Verification items for the finished model (mm, model axes). A direction names the side the tool comes from. Coordinates: 2 decimals unless noted, no trailing zeros. Order: outer loops, then holes, each group sorted by start corner. A loop starts at its lowest first (then second) coordinate and runs counter-clockwise, first axis right, second up. Notation, with made-up numbers: M 66.25,50.25 L 116.25,50.25 A19 ccw 116.25,82.25 Z; hole C 81.5,-26 d11. An arc over 180 degrees is marked long. Return JSON: item names as keys, results as strings.
```python
from build123d import *

# Parameters (mm, degrees)
SKETCH2_W           = 50.8
SKETCH2_H           = 38.1
BOSS_EXTRUDE1_DEPTH = 12.7
FILLET1_R           = 6.35
SKETCH3_R           = 3.81
CUT_EXTRUDE1_DEPTH  = 35.195796525
SKETCH7_W           = 12.7
SKETCH7_H           = 12.7
BOSS_EXTRUDE2_DEPTH = 19.05
SKETCH8_R           = 5.08
CUT_EXTRUDE2_DEPTH  = 25.4
SKETCH9_W           = 6.35
SKETCH9_H           = 38.1
CUT_EXTRUDE3_DEPTH  = 44.45
CUT_EXTRUDE4_REACH  = 52
SKETCH10_W          = 6.35
SKETCH10_H          = 6.35
CHAMFER6_SIZE       = 17.78
CHAMFER6_SIZE_2     = 12.449690029


with BuildPart() as part:
    # Sketch2 → Boss-Extrude1 (new body)
    with BuildSketch(Plane.XY):
        Rectangle(SKETCH2_W, SKETCH2_H)
    extrude(amount=BOSS_EXTRUDE1_DEPTH)

    # Fillet1
    fillet1_edges = [part.edges().sort_by_distance(p)[0] for p in [
        (-25.4, 19.05, 6.35),
        (25.4, 19.05, 6.35),
        (-25.4, -19.05, 6.35),
    ]]
    fillet(fillet1_edges, radius=FILLET1_R)

    # Sketch3 → Cut-Extrude1 (cut, through all)
    with BuildSketch(Plane.XY.offset(12.7)):
        with Locations((-6.35, -10.16)):
            Circle(SKETCH3_R)
    extrude(amount=-CUT_EXTRUDE1_DEPTH, mode=Mode.SUBTRACT)

    # Sketch7 → Boss-Extrude2 (add)
    with BuildSketch(Plane(origin=(25.4, 0, 0), x_dir=(0, 0, -1), z_dir=(1, 0, 0))):
        with Locations((-6.35, 6.35)):
            Rectangle(SKETCH7_W, SKETCH7_H)
    extrude(amount=BOSS_EXTRUDE2_DEPTH)

    # Sketch8 → Cut-Extrude2 (cut)
    with BuildSketch(Plane(origin=(44.45, 0, 0), x_dir=(0, 0, -1), z_dir=(1, 0, 0))):
        with Locations((-6.35, 6.35)):
            Circle(SKETCH8_R)
    extrude(amount=-CUT_EXTRUDE2_DEPTH, mode=Mode.SUBTRACT)

    # Sketch9 → Cut-Extrude3 (cut)
    with BuildSketch(Plane.ZY.offset(25.4)):
        with Locations((3.175, 0)):
            Rectangle(SKETCH9_W, SKETCH9_H)
    extrude(amount=-CUT_EXTRUDE3_DEPTH, mode=Mode.SUBTRACT)

    # Sketch10 → Cut-Extrude4 (cut, up to next)
    with BuildSketch(Plane.ZY.offset(-19.05), mode=Mode.PRIVATE) as cut_extrude4_sk1:
        with Locations((3.175, -15.875)):
            Rectangle(SKETCH10_W, SKETCH10_H)
    cut_extrude4_tool1 = extrude(cut_extrude4_sk1.sketch, amount=-CUT_EXTRUDE4_REACH, mode=Mode.PRIVATE) & part.part
    add(cut_extrude4_tool1.solids().sort_by_distance((19.05, -15.875, 3.175))[0], mode=Mode.SUBTRACT)

    # Chamfer6
    # the kernel refuses this chamfer: 17.78, 12.449690029 mm, written as the material it takes off along each edge
    with BuildSketch(Plane(origin=(25.4, -19.05, -39.567778654), x_dir=(-0.9997533347641299, -0.022209674198457294, 0), z_dir=(0, 0, 1))) as chamfer6_piece_1:
        Polygon((CHAMFER6_SIZE * 0.999753334764, -CHAMFER6_SIZE * 0.0222096741985), (-CHAMFER6_SIZE_2 * 0.0222096741991, -CHAMFER6_SIZE_2 * 0.999753334794), (0, 0), align=None)
    extrude(amount=98.185557309, mode=Mode.SUBTRACT)


solid = part.part
```
Q1. Go/stop test with flat-tipped pins: pin 1 (1.5 mm diameter, centred on y = 4.5, z = 5.5, fed in from -X); pin 2 (3 mm diameter, centred on y = 2.5, z = 2.5, fed in from -X); pin 3 (19 mm diameter, centred on x = -3, y = 4, fed in from -Z); pin 4 (4 mm diameter, centred on x = 34.5, z = 7, fed in from -Y). Record where each tip stops, or that it passes through.
Values:
{"pin 1": "through", "pin 2": "x = 19.05", "pin 3": "z = 6.35", "pin 4": "y = 0"}
Q2. Material ranges on line 1 along Y through (x, z) = (31.5, 6.35); line 2 along X through (y, z) = (-3, 2), recorded low to high.
Values:
{"line 1": "0 to 1.27, 11.43 to 12.7", "line 2": "19.05 to 25.4"}
Q3. Cross-section at B-B, the plane x = -6.35. Record the boundary of the cut face in (y, z), and give its area (3 significant figures).
Values:
{"outline": "M -19.05,6.35 L -13.97,6.35 L -13.97,12.7 L -19.05,12.7 Z; M -6.35,6.35 L 19.05,6.35 L 19.05,12.7 L -6.35,12.7 Z", "area": "194 mm^2"}
Q4. Tool access check on faces 4 (the face through (35, 0, 6)), 5 (the face through (19.05, 6, 8)), 6 (the face through (35, 12.7, 6)), 7 (the face through (-3, 0, 6.35)). Record the directions out of +Z, -Z, +X, -X, +Y, -Y that give a thin tool (end or side, any length) a straight path to the whole face; none if there is none.
Values:
{"face 4": "+Z, -Z, +X, -Y", "face 5": "+X", "face 6": "+Z, -Z, +X, +Y", "face 7": "-Z, -X, +Y, -Y"}
Q5. Cross-section at C-C, the plane z = 3.5. Record the boundary of the cut face in (x, y), and give its area (3 significant figures).
Values:
{"outline": "M 19.05,-11.05 L 25.4,-6.6 L 25.4,0 L 44.45,0 L 44.45,2.14 L 19.05,2.14 Z; M 19.05,10.56 L 44.45,10.56 L 44.45,12.7 L 25.4,12.7 A6.35 ccw 19.05,19.05 Z", "area": "197 mm^2"}
Q6. Cross-section at D-D, the plane z = 10.5. Record the boundary of the cut face in (x, y), and give its area (3 significant figures).
Values:
{"outline": "M -25.4,-12.7 A6.35 ccw -19.05,-19.05 L 7.62,-19.05 L 25.4,-6.6 L 25.4,0 L 44.45,0 L 44.45,3.42 L 19.05,3.42 L 19.05,9.28 L 44.45,9.28 L 44.45,12.7 L 25.4,12.7 A6.35 ccw 19.05,19.05 L -19.05,19.05 A6.35 ccw -25.4,12.7 Z; hole C -6.35,-10.16 d7.62", "area": "1,850 mm^2"}
Q7. Cross-section at A-A, the plane y = 6.35. Record the boundary of the cut face in (x, z).
Values:
{"outline": "M -25.4,6.35 L 19.05,6.35 L 19.05,11.43 L 44.45,11.43 L 44.45,12.7 L -25.4,12.7 Z; M 19.05,0 L 44.45,0 L 44.45,1.27 L 19.05,1.27 Z"}
Q8. Draft check along Z on faces 1 (the face through (19.05, 4, 1)), 2 (the face through (31.928, 7.876, 1.505)), 3 (the face through (1, 0, 12.7)). Enter one of: pulls with the +Z half, pulls with the -Z half, needs draft (parallel to the pull), parting line crosses it, or undercut.
Values:
{"face 1": "needs draft", "face 2": "undercut", "face 3": "pulls with the +Z half"}
